```python
from build123d import *

# Parameters (mm, degrees)
SKETCH_6_W                = 22
SKETCH_6_H                = 4.5
CUT_EXTRUDE_4_DEPTH       = 5
CUT_EXTRUDE_11_DEPTH      = 189.679622641
CUT_EXTRUDE_11_DEPTH_BACK = 189.679622641
SKETCH_6_3_W              = 50
SKETCH_6_3_H              = 5
SKETCH_16_R               = 6
CUT_EXTRUDE_10_DEPTH      = 189.679622641
PATTERN_CIRCULAR_1_COUNT  = 4
CHAMFER_3_SIZE            = 2


with BuildPart() as part:
    # Sketch 1 → Revolve 1 (revolve)
    with BuildSketch(Plane.XY, mode=Mode.PRIVATE) as revolve_1_sk:
        Polygon((0, 10), (0, 22.5), (60, 22.5), (60, 40), (125, 40), (125, 17), (180, 17), (180, 10), align=None)
    revolve(revolve_1_sk.sketch.rotate(Axis((0, 0, 0), (-1, 0, 0)), 90), axis=Axis((0, 0, 0), (-1, 0, 0)))

    # Sketch 6 → Cut-Extrude 4 (cut, symmetric)
    with BuildSketch(Plane.XY):
        with Locations((159, 14.75)):
            Rectangle(SKETCH_6_W, SKETCH_6_H)
    extrude(amount=CUT_EXTRUDE_4_DEPTH, both=True, mode=Mode.SUBTRACT)

    # Sketch 6_3 → Cut-Extrude 11 (cut, two sides: drawn at the far end of the back side and taken through both)
    with BuildSketch(Plane.XY.offset(-CUT_EXTRUDE_11_DEPTH_BACK)):
        with Locations((25, 20)):
            Rectangle(SKETCH_6_3_W, SKETCH_6_3_H)
    extrude(amount=CUT_EXTRUDE_11_DEPTH + CUT_EXTRUDE_11_DEPTH_BACK, mode=Mode.SUBTRACT)

    # Sketch 16 → Cut-Extrude 10 (cut, symmetric)
    with BuildSketch(Plane(origin=(0, 0, 0), x_dir=(1, 0, 0), z_dir=(0, 1, 0))):
        with Locations(Location((92.5, 0, 0), (0, 0, 270))):
            Circle(SKETCH_16_R)
    cut_extrude_10 = extrude(amount=CUT_EXTRUDE_10_DEPTH, both=True, mode=Mode.SUBTRACT)

    # Pattern Circular 1: Cut-Extrude 10 ×4 about axis
    pattern_circular_1_axis = Axis((0, 0, 0), (1, 0, 0))
    for i in range(1, PATTERN_CIRCULAR_1_COUNT):
        add(cut_extrude_10.rotate(pattern_circular_1_axis, i * 360 / PATTERN_CIRCULAR_1_COUNT), mode=Mode.SUBTRACT)

    # Chamfer 3
    chamfer_3_edges = [part.edges().sort_by_distance(p)[0] for p in [
        (0, -20.303300859, 9.696699141),
        (180, 0, 17),
        (125, 0, 40),
        (60, 0, 40),
    ]]
    chamfer(chamfer_3_edges, length=CHAMFER_3_SIZE)


solid = part.part
```
The model under review builds one solid part; all positions refer to its coordinate system, in mm. A direction names the side the tool comes from. Give positions to 0.01 mm unless a question says otherwise; leave off trailing zeros. Write each loop counter-clockwise with the first axis right and the second up, starting at its lowest first coordinate (ties: lowest second). Pieces come first, ordered by that corner, then holes.
(1) To check wall thickness, follow L1, parallel to X at y = 15, z = 0; L2, parallel to X at y = 28, z = 0; L3, parallel to X at y = -15, z = 0. State the ranges of each line that lie inside material, in increasing order.
(2) For P1, Ø7, axis at x = 92.5, y = 0, coming from the +Z side; P2, Ø14, axis at x = 92.5, z = 0, coming from the +Y side; P3, Ø8, axis at x = 88, y = 27.5, coming from the -Z side; P4, Ø1.5, axis at y = 19, z = 0, coming from the -X side, all flat-tipped, find the tip position at first contact; note any pin that passes through.
(3) Consider section D-D, the plane x = 92.5. Give the boundary of the cut face in (y, z), and give its area (3 significant figures).
(4) Consider section A-A, the plane y = 0. Give the number of separate pieces and of enclosed holes in the cut face, and give its area (3 significant figures).
(5) Consider section B-B, the plane x = 158. Give the boundary of the cut face in (y, z), and give its area (3 significant figures).
(6) The part is to be moulded in two halves that separate along Y. For faces 4 (the cylindrical face through (92.927, 35.487, -18.458)), 5 (the cylindrical face through (88.74, -6.76, 7.37)), 6 (the cylindrical face through (98.45, 0.78, 24.22)), 7 (the flat face through (0, -10.2, -0.3)), say which applies: released by +Y, released by -Y, zero draft, split by the parting line, or undercut.
(7) Tool access review of faces 1 (the flat face through (159, 14, 5)), 2 (the flat face through (50, 19, 0)), 3 (the cylindrical face through (151.871, -16.855, 2.213)): name each direction out of +Z, -Z, +X, -X, +Y, -Y from which nothing blocks a thin tool from reaching the whole face with its end or side.
Returned:
1. L1: x = 0 to 86.5, 98.5 to 148, 170 to 180
1. L2: x = 60 to 86.5, 98.5 to 125
1. L3: x = 0 to 86.5, 98.5 to 180
2. P1: passes through
2. P2: stops at y = 40
2. P3: stops at z = -32.37
2. P4: stops at x = 50
3. outline: (-39.55, -6) arc R40 ccw to (-6, -39.55) - (-6, -8) arc R10 cw to (-8, -6) - close; (-39.55, 6) - (-8, 6) arc R10 cw to (-6, 8) - (-6, 39.55) arc R40 ccw to start; (6, -39.55) arc R40 ccw to (39.55, -6) - (8, -6) arc R10 cw to (6, -8) - close; (6, 8) arc R10 cw to (8, 6) - (39.55, 6) arc R40 ccw to (6, 39.55) - close
3. area: 3,250 mm2
4. separate pieces: 4
4. enclosed holes: 0
4. area: 5,430 mm2
5. outline: (12.5, -5) - (12.5, 5) - (16.25, 5) arc R17 ccw (long way) to (16.25, -5) - close; hole circle Ø20 at (0, 0)
5. area: 551 mm2
6. face 4: split by the parting line
6. face 5: undercut
6. face 6: undercut
6. face 7: zero draft
7. face 1: +Y
7. face 2: +Z, -Z, -X, +Y
7. face 3: +X
